Autodesk Inventor part; units mm, degrees
ref_plane "Mitad" through (1, 20, 0) normal (0, 1, 0) x (1, 0, 0)
ref_plane "YZ Plane" through (0, 0, 0) normal (1, 0, 0) x (0, 1, 0)
ref_plane "XZ Plane" through (0, 0, 0) normal (0, 1, 0) x (-1, 0, 0)
sketch "Boceto1" plane through (0, 0, 0) normal (0, 0, 1) x (1, 0, 0)
  line L0 (0, 0) -> (200, 0)
  line L1 (200, 0) -> (200, 40)
  line L2 (200, 40) -> (0, 40)
  line L3 (0, 40) -> (0, 0)
  dimension "d0" = 200
  dimension "d1" = 40
extrude "Base" add sketch "Boceto1" along normal blind 2
sketch "Boceto2" plane through (0, 0, 2) normal (0, 0, 1) x (1, 0, 0)
  line L0 (200, 40) -> (200, 0)
  line L1 (200, 22) -> (2, 22)
  line L2 (2, 22) -> (2, 18)
  line L3 (2, 18) -> (200, 18)
  line L4 (200, 18) -> (200, 22)
  point P0 (0, 40)
  point P1 (200, 20)
  dimension "d4" = 4
  dimension "d5" = 2
extrude "Canal" cut sketch "Boceto2" against normal blind 1
sketch "Boceto3" plane through (0, 0, 2) normal (0, 0, 1) x (1, 0, 0)
  line L0 (2, 22) -> (200, 22)
  line L1 (200, 40) -> (200, 22)
  line L2 (0, 40) -> (200, 40)
  line L3 (0, 0) -> (0, 40)
  line L4 (200, 0) -> (0, 0)
  line L5 (200, 18) -> (200, 0)
  line L6 (198, 38) -> (2, 38)
  line L7 (2, 38) -> (2, 2)
  line L8 (2, 2) -> (198, 2)
  line L9 (198, 2) -> (198, 9)
  line L10 (198, 9) -> (200, 9)
  line L11 (198, 38) -> (198, 31)
  line L12 (198, 31) -> (200, 31)
  dimension "d8" = 2
  dimension "d9" = 2
  dimension "d10" = 2
  dimension "d11" = 2
  dimension "d12" = 2
  dimension "d33" = 7
  dimension "d34" = 7
extrude "Paredes" add sketch "Boceto3" along normal blind 7 contours L7 L8 L9 L10 L5 L4 L3 L2 L1 L12 L11 L6
ref_plane "Mitad" through (1, 20, 0) normal (0, 1, 0) x (1, 0, 0)
sketch "Boceto4" plane through (0, 0, 2) normal (0, 0, 1) x (1, 0, 0)
  line L0 (200, 0) -> (0, 0)
  point P0 (49, 4.3)
  point P1 (151, 4.3)
  dimension "d36" = 4.3
  dimension "d37" = 4.3
hole "Hole1" at (49, 4.3, 2) at (151, 4.3, 2) direction (0, 0, -1) diameter 1 end through all
sketch "Boceto5" plane through (0, 0, 2) normal (0, 0, 1) x (1, 0, 0)
  line L0 (2, 38) -> (2, 22)
  line L1 (198, 38) -> (2, 38)
  line L2 (136, 35) -> (64, 35)
  line L3 (64, 35) -> (66, 33)
  line L4 (66, 33) -> (134, 33)
  line L5 (134, 33) -> (136, 35)
  line L6 (198, 31) -> (198, 38)
  point P0 (0, 0)
  dimension "d23" = 2
  dimension "d24" = 2
  dimension "d25" = 3
  dimension "d26" = 62
  dimension "d35" = 62
extrude "Extrusión4" add sketch "Boceto5" along normal blind 2.5
sketch "Boceto6" plane through (0, 0, 4.5) normal (0, 0, 1) x (1, 0, 0)
  line L0 (64, 35) -> (136, 35)
  line L1 (134, 33) -> (66, 33)
  line L2 (96, 35) -> (104, 35)
  line L3 (104, 35) -> (104, 33)
  line L4 (104, 33) -> (96, 33)
  line L5 (96, 33) -> (96, 35)
  point P0 (0, 0)
  point P1 (100, 35)
  dimension "d30" = 8
extrude "Extrusión5" add sketch "Boceto6" along normal blind 2
mirror "Simetría1" about plane through (1, 20, 0) normal (0, 1, 0) of "Extrusión4", "Extrusión5"
properties part number "Base"
Could you check a few things on this model? Use its own coordinates, in mm. A direction names the side the tool comes from. Give positions to 0.01 mm unless a question says otherwise; leave off trailing zeros. Loops run counter-clockwise (first coordinate to the right, second up) from the corner with the lowest first, then second, coordinate; pieces in that order, holes last. Notation, with made-up numbers: (53, -35.75) - (95, -35.75) arc R18 cw to (95, -4.75) - close; hole circle Ø9 at (85.5, 57). An arc over 180 degrees is marked (long way). Answer in a Markdown table with one row per item. Add a question column.
Q1. We'd pull the mould along Y, two halves only. Please class faces 1 (the face through (101, 0, 4)), 2 (the face through (100, 10, 2)), 3 (the face through (99, 20, 0)): +Y half, -Y half, draft (parallel to the pull), parting line (faces both ways), or undercut.
Q2. Which directions (+Z, -Z, +X, -X, +Y, -Y) give clear straight access to the entire face, cutting with the end or side of a thin tool? Please do faces 4 (the face through (101, 35, 3)), 5 (the face through (100, 20, 1)), 6 (the face through (200, 19.7, 0.4)).
Q3. Please list where these lines run through material, in increasing order: L1, parallel to X at y = 4.3, z = 0.4; L2, parallel to Y at x = 151, z = 1.2; L3, parallel to Y at x = 60, z = 8. Write a range as from..to.
Q4. If we section it at B-B (y = 15.5): List the corners of the cut face in (x, z) for me.
Q5. If we section it at A-A (x = 22): List the corners of the cut face in (y, z) for me.
Q6. For pin 1 (3 mm diameter, centred on y = 24.5, z = 5.5, fed in from +X); pin 2 (2 mm diameter, centred on x = 77, y = 6.5, fed in from +Z); pin 3 (2 mm diameter, centred on x = 148, y = 19.5, fed in from +Z), each with a flat end and sliding along its axis, tell me the tip position at first contact or that it passes through.
The answers:
| question | item | result |
|---|---|---|
| 1 | face 1 | -Y half |
| 1 | face 2 | undercut |
| 1 | face 3 | draft |
| 2 | face 4 | +Z |
| 2 | face 5 | +Z, +X |
| 2 | face 6 | +Z, -Z, +X, +Y, -Y |
| 3 | L1 | x = 0..48.5, 49.5..150.5, 151.5..200 |
| 3 | L2 | y = 0..3.8, 4.8..18, 22..40 |
| 3 | L3 | y = 0..2, 38..40 |
| 4 | outline | (0, 0) - (200, 0) - (200, 2) - (2, 2) - (2, 9) - (0, 9) - close |
| 5 | outline | (0, 0) - (40, 0) - (40, 9) - (38, 9) - (38, 2) - (22, 2) - (22, 1) - (18, 1) - (18, 2) - (2, 2) - (2, 9) - (0, 9) - close |
| 6 | pin 1 | stops at x = 2 |
| 6 | pin 2 | stops at z = 4.5 |
| 6 | pin 3 | stops at z = 1 |
